Drawing for the job (mm, zero at the part's lowest x, y, z). A direction names the side the tool comes from. Give positions to 0.01 mm unless a question says otherwise; leave off trailing zeros. Loops run counter-clockwise (first coordinate to the right, second up) from the corner with the lowest first, then second, coordinate; pieces in that order, holes last. Notation, with made-up numbers: (61.25, 18) -> (91.25, 18) arc R13 cw to (91.25, 42) -> close; hole circle Ø2 at (20.5, -20). An arc over 180 degrees is marked (long way). Answer in a Markdown table with one row per item. Add a question column.
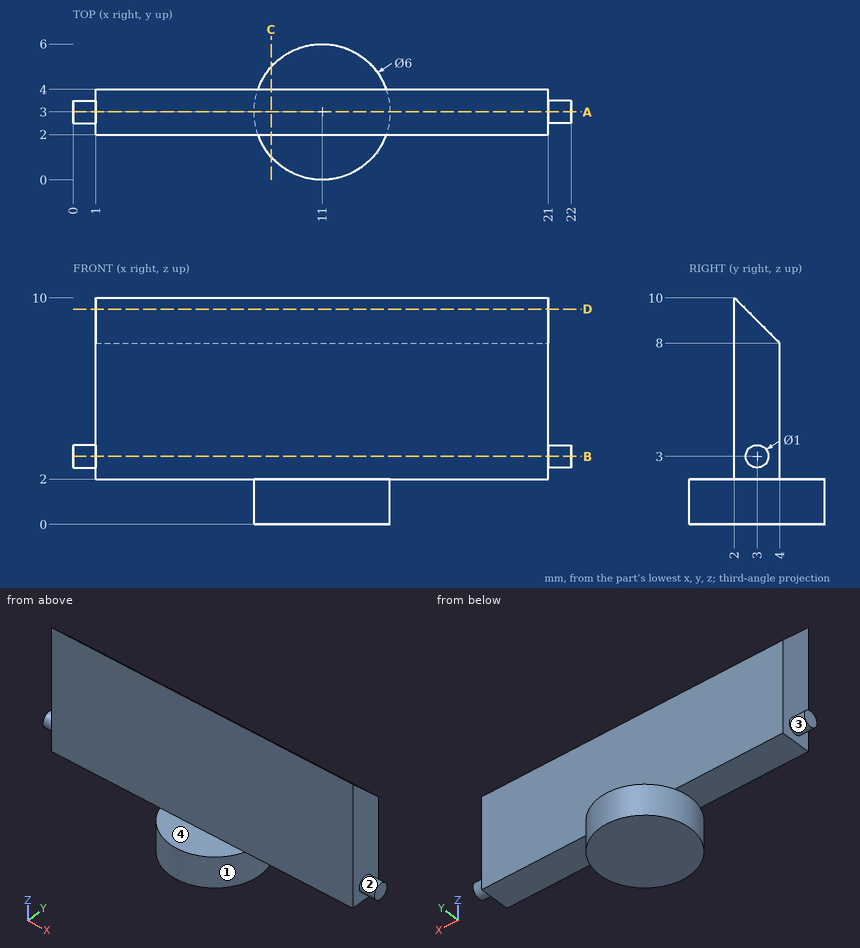
(1) Flat gauge pins, fed straight in: pin 1 Ø0.6 at (x, y) = (11.5, 5) entering from +Z; pin 2 Ø2 at (y, z) = (0.5, 1.5) entering from +X; pin 3 Ø1 at (x, y) = (4.5, 3) entering from -Z. Where does each tip first touch, or does it go through?
(2) 3-axis set-ups, long thin cutter, end or side, ignore diameter. For the marked faces 1, 2, 3 and 4: which of +Z, -Z, +X, -X, +Y, -Y reach the whole face in a straight line?
(3) Wall check: line 1 along Y through (x, z) = (3, 9.5); line 2 along Y through (x, z) = (2.75, 2.5); line 3 along X through (y, z) = (3.75, 5.75). Give the ranges that are in metal, low to high. Write a range as from..to.
(4) Saw through at B-B, the plane z = 3. List the corners of the cut face in (x, y), then the cut area to 3 significant figures.
(5) Saw through at A-A, the plane y = 3. List the corners of the cut face in (x, z), then the cut area to 3 significant figures.
(6) Saw through at D-D, the plane z = 9.5. List the corners of the cut face in (x, y).
(7) Saw through at C-C, the plane x = 8.75. List the corners of the cut face in (y, z).
Worked answers:
| question | item | result |
|---|---|---|
| 1 | pin 1 | z = 2 |
| 1 | pin 2 | x = 13.6 |
| 1 | pin 3 | z = 2 |
| 2 | face 1 | -Z |
| 2 | face 2 | +X |
| 2 | face 3 | -X |
| 2 | face 4 | +Z, +X, -X, -Y |
| 3 | line 1 | 2..2.5 |
| 3 | line 2 | 2..4 |
| 3 | line 3 | 1..21 |
| 4 | outline | (0, 2.5) -> (1, 2.5) -> (1, 2) -> (21, 2) -> (21, 2.5) -> (22, 2.5) -> (22, 3.5) -> (21, 3.5) -> (21, 4) -> (1, 4) -> (1, 3.5) -> (0, 3.5) -> close |
| 4 | area | 42.0 mm^2 |
| 5 | outline | (0, 2.5) -> (1, 2.5) -> (1, 2) -> (8, 2) -> (8, 0) -> (14, 0) -> (14, 2) -> (21, 2) -> (21, 2.5) -> (22, 2.5) -> (22, 3.5) -> (21, 3.5) -> (21, 9) -> (1, 9) -> (1, 3.5) -> (0, 3.5) -> close |
| 5 | area | 154 mm^2 |
| 6 | outline | (1, 2) -> (21, 2) -> (21, 2.5) -> (1, 2.5) -> close |
| 7 | outline | (1.02, 0) -> (4.98, 0) -> (4.98, 2) -> (4, 2) -> (4, 8) -> (2, 10) -> (2, 2) -> (1.02, 2) -> close |
